```python
from build123d import *

# Parameters (mm, degrees)
SKETCH1_W           = 27.6032
SKETCH1_H           = 35.3248
SKETCH1_W_2         = 25.6032
SKETCH1_H_2         = 33.3248
MAINCASING_DEPTH    = 12.93
SKETCH2_W           = 6.35
SKETCH2_H           = 9.525
SKETCH2_R           = 1.4732
MOUNTINGTABS_DEPTH  = 1.5875
SKETCH3_W           = 3.683
SKETCH3_H           = 7.112
SKETCH3_W_2         = 4.572
SKETCH3_H_2         = 4.572
SKETCH3_R           = 1.1303
BOSS_EXTRUDE3_DEPTH = 12.93
SKETCH4_W           = 27.6032
SKETCH4_H           = 35.3248
SKETCH4_W_2         = 25.6032
SKETCH4_H_2         = 33.3248
BOSS_EXTRUDE4_DEPTH = 1.6002
SKETCH5_R           = 1.1303
UPPERHOLES_DEPTH    = 38.848662667
SKETCH6_W           = 25.6032
SKETCH6_H           = 1
BOSS_EXTRUDE5_DEPTH = 12.93
SKETCH7_W           = 27.6032
SKETCH7_H           = 1
CUT_EXTRUDE2_DEPTH  = 38.848662667


with BuildPart() as part:
    # Sketch1 → mainCasing (new body)
    with BuildSketch(Plane(origin=(0, 0, 0), x_dir=(1, 0, 0), z_dir=(0, 1, 0))):
        with Locations((2.873828571, -8.628742857)):
            Rectangle(SKETCH1_W, SKETCH1_H)
        with Locations((2.873828571, -8.628742857)):
            Rectangle(SKETCH1_W_2, SKETCH1_H_2, mode=Mode.SUBTRACT)
    extrude(amount=-MAINCASING_DEPTH)

    # Sketch2 → mountingTabs (add)
    # profile 1 of 2: a face of its own
    with BuildSketch(Plane.XZ.offset(12.93)):
        with Locations((-14.102771429, 8.628742857)):
            Rectangle(SKETCH2_W, SKETCH2_H)
        with Locations(Location((-14.102771429, 8.628742857, 0), (0, 0, 270))):
            Circle(SKETCH2_R, mode=Mode.SUBTRACT)
    # profile 2 of 2: a face of its own
    with BuildSketch(Plane.XZ.offset(12.93)):
        with Locations((19.850428571, 8.628742857)):
            Rectangle(SKETCH2_W, SKETCH2_H)
        with Locations(Location((19.850428571, 8.628742857, 0), (0, 0, 270))):
            Circle(SKETCH2_R, mode=Mode.SUBTRACT)
    extrude(amount=-MOUNTINGTABS_DEPTH)

    # Sketch3 → Boss-Extrude3 (add)
    # profile 1 of 4: a face of its own
    with BuildSketch(Plane(origin=(0, 0, 0), x_dir=(1, 0, 0), z_dir=(0, 1, 0))):
        with Locations((-8.086271429, 4.477657143)):
            Rectangle(SKETCH3_W, SKETCH3_H)
    # profile 2 of 4: a face of its own
    with BuildSketch(Plane(origin=(0, 0, 0), x_dir=(1, 0, 0), z_dir=(0, 1, 0))):
        with Locations((13.833928571, 4.477657143)):
            Rectangle(SKETCH3_W, SKETCH3_H)
    # profile 3 of 4: a face of its own
    with BuildSketch(Plane(origin=(0, 0, 0), x_dir=(1, 0, 0), z_dir=(0, 1, 0))):
        with Locations((-7.641771429, -19.703142857)):
            Rectangle(SKETCH3_W_2, SKETCH3_H_2)
        with Locations(Location((-7.235371429, -19.703142857, 0), (0, 0, 270))):
            Circle(SKETCH3_R, mode=Mode.SUBTRACT)
    # profile 4 of 4: a face of its own
    with BuildSketch(Plane(origin=(0, 0, 0), x_dir=(1, 0, 0), z_dir=(0, 1, 0))):
        with Locations((13.389428571, -19.703142857)):
            Rectangle(SKETCH3_W_2, SKETCH3_H_2)
        with Locations(Location((12.983028571, -19.703142857, 0), (0, 0, 270))):
            Circle(SKETCH3_R, mode=Mode.SUBTRACT)
    extrude(amount=-BOSS_EXTRUDE3_DEPTH)

    # Sketch4 → Boss-Extrude4 (add)
    with BuildSketch(Plane(origin=(0, 0, 0), x_dir=(1, 0, 0), z_dir=(0, 1, 0))):
        with Locations((2.873828571, -8.628742857)):
            Rectangle(SKETCH4_W, SKETCH4_H)
        with Locations((2.873828571, -8.628742857)):
            Rectangle(SKETCH4_W_2, SKETCH4_H_2, mode=Mode.SUBTRACT)
    extrude(amount=BOSS_EXTRUDE4_DEPTH)

    # Sketch5 → upperHoles (cut, through all)
    with BuildSketch(Plane.XZ.offset(12.93)):
        with Locations((-7.235371429, -4.731657143)):
            Circle(SKETCH5_R)
        with Locations((12.983028571, -4.731657143)):
            Circle(SKETCH5_R)
    extrude(amount=-UPPERHOLES_DEPTH, mode=Mode.SUBTRACT)

    # Sketch6 → Boss-Extrude5 (add)
    with BuildSketch(Plane.XZ.offset(12.93)):
        with Locations((2.873828571, 12.786342857)):
            Rectangle(SKETCH6_W, SKETCH6_H)
    extrude(amount=-BOSS_EXTRUDE5_DEPTH)

    # Sketch7 → Cut-Extrude2 (cut, through all)
    with BuildSketch(Plane.XZ.offset(12.93)):
        with Locations((2.873828571, 25.791142857)):
            Rectangle(SKETCH7_W, SKETCH7_H)
    extrude(amount=-CUT_EXTRUDE2_DEPTH, mode=Mode.SUBTRACT)


solid = part.part
```
For this review, take the finished solid that the model builds, in its own axes (mm). A direction names the side the tool comes from. Give positions to 0.01 mm unless a question says otherwise; leave off trailing zeros. Order: outer loops, then holes, each group sorted by start corner. A loop starts at its lowest first (then second) coordinate and runs counter-clockwise, first axis right, second up.
1) For faces 4 (the face through (-14, -12, 3.866)), 5 (the face through (3, 0, 13)), 6 (the face through (11.103, -6, 20)), 7 (the face through (3, -7, 12.286)), list the 3-axis set-ups (+Z, -Z, +X, -X, +Y, -Y) from which the entire face can be reached by the end or side of a thin tool; tool diameter is ignored.
2) The part is to be moulded in two halves that separate along X. For faces 1 (the face through (23.025, -12, 9)), 2 (the face through (-12.7, -11.342, 7.6)), 3 (the face through (14, -6, -0.922)), say which applies: released by +X, released by -X, zero draft, split by the parting line, or undercut.
3) Insertion check: pin 1 (0.8 mm diameter, centred on x = 19.5, y = -12.5, fed in from +Z); pin 2 (4 mm diameter, centred on y = -6.5, z = 7.5, fed in from -X); pin 3 (1.7 mm diameter, centred on x = 20.5, y = -12.5, fed in from -Z); pin 4 (3 mm diameter, centred on x = -3, z = -5, fed in from +Y). Each pin has a flat end and moves straight along its axis. Give the tip position at first contact, or say it passes through.
4) Take a section at C-C (x = 13.5). Give the boundary of the cut face in (y, z).
5) Wall thickness on line 1 (Z direction, x = -8.5, y = -11.25); line 2 (X direction, y = -12.25, z = -3.5); line 3 (Z direction, x = 14, y = -1): over which ranges is each line inside the solid? List them lowest first.
6) Take a section at A-A (x = -4.5). Give the boundary of the cut face in (y, z), then the cut area to 3 significant figures.
7) Take a section at B-B (z = 18). Give the boundary of the cut face in (x, y).
8) Take a section at D-D (y = -7.75). State how many separate pieces and enclosed holes the cut face has, then the cut area to 3 significant figures.
Derived:
1. face 4: -Z, -X, +Y, -Y
1. face 5: +Z, +Y
1. face 6: +Z, +Y, -Y
1. face 7: +Y, -Y
2. face 1: released by +X
2. face 2: zero draft
2. face 3: undercut
3. pin 1: stops at z = 13.39
3. pin 2: stops at x = -10.93
3. pin 3: stops at z = 3.87
3. pin 4: passes through
4. outline: (-12.93, -9.03) - (1.6, -9.03) - (1.6, -8.03) - (0, -8.03) - (0, -5.74) - (-12.93, -5.74) - close; (-12.93, -3.73) - (0, -3.73) - (0, -0.92) - (-12.93, -0.92) - close; (-12.93, 12.29) - (0, 12.29) - (0, 13.29) - (-12.93, 13.29) - close; (-12.93, 17.42) - (0, 17.42) - (0, 18.7) - (-12.93, 18.7) - close; (-12.93, 20.71) - (0, 20.71) - (0, 21.99) - (-12.93, 21.99) - close
5. line 1: z = -9.03 to -0.92, 12.29 to 13.29, 17.42 to 21.99
5. line 2: x = -10.93 to -6.24, 11.99 to 16.68
5. line 3: z = -9.03 to -5.22, -4.24 to -0.92, 12.29 to 13.29, 17.42 to 19.21, 20.2 to 21.99
6. outline: (-12.93, -9.03) - (1.6, -9.03) - (1.6, -8.03) - (-12.93, -8.03) - close; (-12.93, 12.29) - (0, 12.29) - (0, 13.29) - (-12.93, 13.29) - close
6. area: 27.5 mm2
7. outline: (-10.93, -12.93) - (-5.36, -12.93) - (-5.36, 0) - (-9.93, 0) - (-9.93, 1.6) - (-10.93, 1.6) - close; (11.1, -12.93) - (16.68, -12.93) - (16.68, 1.6) - (15.68, 1.6) - (15.68, 0) - (11.1, 0) - close
8. separate pieces: 1
8. enclosed holes: 3
8. area: 198 mm2
